Could you check a few things on this model? Use its own coordinates, in mm. A direction names the side the tool comes from. Coordinates: 2 decimals unless noted, no trailing zeros. Write each loop counter-clockwise with the first axis right and the second up, starting at its lowest first coordinate (ties: lowest second). Pieces come first, ordered by that corner, then holes.
```python
from build123d import *

# Parameters (mm, degrees)
BOSS_EXTRUDE1_DEPTH = 76.2
SKETCH3_R           = 9.525
CUT_EXTRUDE1_DEPTH  = 151.268426491


with BuildPart() as part:
    # Sketch2 → Boss-Extrude1 (new body)
    with BuildSketch(Plane.XY):
        Polygon((25.4, 25.4), (25.4, 12.7), (76.2, 12.7), (76.2, 25.4), (127, 25.4), (127, 0), (0, 0), (0, 25.4), align=None)
    extrude(amount=-BOSS_EXTRUDE1_DEPTH)

    # Sketch3 → Cut-Extrude1 (cut, through all)
    with BuildSketch(Plane(origin=(0, 25.4, 0), x_dir=(1, 0, 0), z_dir=(0, 1, 0))):
        with Locations(Location((101.6, 38.1, 0), (0, 0, 270))):
            Circle(SKETCH3_R)
    extrude(amount=-CUT_EXTRUDE1_DEPTH, mode=Mode.SUBTRACT)


solid = part.part
```
1. I want a section at C-C on y = 2.5. Please give me the cut outline in (x, z) (3 decimals), plus the area to 3 significant figures.
Verdict:
outline: (0, -76.2) - (127, -76.2) - (127, 0) - (0, 0) - close; hole circle Ø19.05 at (101.6, -38.1)
area: 9,390 mm2
2. I want a section at B-B on z = -38.1. Please give me the cut outline in (x, y) (3 decimals), plus the area to 3 significant figures.
Verdict:
outline: (0, 0) - (92.075, 0) - (92.075, 25.4) - (76.2, 25.4) - (76.2, 12.7) - (25.4, 12.7) - (25.4, 25.4) - (0, 25.4) - close; (111.125, 0) - (127, 0) - (127, 25.4) - (111.125, 25.4) - close
area: 2,100 mm2
3. For pin 1 (17 mm diameter, centred on x = 101.6, z = -38.1, fed in from +Y); pin 2 (2 mm diameter, centred on x = 28, z = -56.5, fed in from +Y), each with a flat end and sliding along its axis, tell me the tip position at first contact or that it passes through.
Verdict:
pin 1: passes through
pin 2: stops at y = 12.7
4. Please list where these lines run through material, in increasing order: line 1 along X through (y, z) = (14.75, -38.1) (3 decimals); line 2 along X through (y, z) = (14.25, -27); line 3 along X through (y, z) = (9.5, -38.1) (3 decimals).
Verdict:
line 1: x = 0 to 25.4, 76.2 to 92.075, 111.125 to 127
line 2: x = 0 to 25.4, 76.2 to 127
line 3: x = 0 to 92.075, 111.125 to 127
5. If we mould it in two halves opening along Z, with no side actions, what happens to faces 3 (the face through (64, 10, -76.2)), 4 (the face through (64, 10, 0)), 5 (the face through (25.4, 19, -38)), 6 (the face through (104.461, 12.878, -29.015))? For each: pulls with the +Z half, pulls with the -Z half, needs draft (parallel to the pull), parting line crosses it, or undercut.
Verdict:
face 3: pulls with the -Z half
face 4: pulls with the +Z half
face 5: needs draft
face 6: undercut
6. On a 3-axis mill with a long thin cutter (end or side, diameter ignored), from which of +Z, -Z, +X, -X, +Y, -Y can I reach the whole of each face in a straight line? I mean faces 1 (the face through (0, 13, -38)), 2 (the face through (76.2, 19, -38)). Say none if no direction works.
Verdict:
face 1: +Z, -Z, -X, +Y, -Y
face 2: +Z, -Z, +Y
7. I want a section at D-D on z = -66. Please give me the cut outline in (x, y).
Verdict:
outline: (0, 0) - (127, 0) - (127, 25.4) - (76.2, 25.4) - (76.2, 12.7) - (25.4, 12.7) - (25.4, 25.4) - (0, 25.4) - close
8. I want a section at A-A on x = 101.6. Please give me the cut outline in (y, z) (3 decimals).
Verdict:
outline: (0, -76.2) - (25.4, -76.2) - (25.4, -47.625) - (0, -47.625) - close; (0, -28.575) - (25.4, -28.575) - (25.4, 0) - (0, 0) - close
